```python
from build123d import *

# Parameters (mm, degrees)
PROFILE_EXTRUDE_DEPTH               = 23
PROFILE_EXTRUDE_DEPTH_BACK          = 23
PROFILE_SHELL_T                     = -3
CUFF_JOINT_PIN_SKETCH_R             = 7.5
CUFF_JOIN_PIN_EXTRUDE_DEPTH         = 43
HYDRAULIC_ARM_HOLES_SKETCH_R        = 5
HYDRAULIC_ARM_HOLES_EXTRUDE_1_DEPTH = 3
HYDRAULIC_START                     = -43
HYDRAULIC_ARM_HOLES_SKETCH_2_R      = 5
HYDRAULIC_ARM_HOLES_EXTRUDE_2_DEPTH = 3
HOLES_TABS_FILLET_R                 = 5


with BuildPart() as part:
    # Profile Sketch → Profile Extrude (new, two sides: drawn at the far end of the back side and taken through both)
    with BuildSketch(Plane(origin=(0, 0, 0), x_dir=(0, 0, -1), z_dir=(1, 0, 0)).offset(-PROFILE_EXTRUDE_DEPTH_BACK)):
        with BuildLine():
            Line((-80, 23), (100, 23))
            Line((100, 23), (100, 0))
            ThreePointArc((100, 0), (93.263455967, -16.263455967), (77, -23))
            Line((77, -23), (-100, -23))
            Line((-100, -23), (-100, 3))
            ThreePointArc((-100, 3), (-94.142135624, 17.142135624), (-80, 23))
        make_face()
    extrude(amount=PROFILE_EXTRUDE_DEPTH + PROFILE_EXTRUDE_DEPTH_BACK)

    # Profile Shell
    profile_shell_openings = [part.faces().sort_by_distance(p)[0] for p in [
        (0, 11.5, -100),
        (0, -16.263455967, -93.263455967),
        (0, -23, 11.5),
    ]]
    offset(amount=PROFILE_SHELL_T, openings=profile_shell_openings, kind=Kind.INTERSECTION)

    # Cuff Joint Pin Sketch → Cuff Join Pin Extrude (add)
    with BuildSketch(Plane(origin=(23, 0, 0), x_dir=(0, 0, -1), z_dir=(1, 0, 0))):
        with Locations((77, 0)):
            Circle(CUFF_JOINT_PIN_SKETCH_R)
    extrude(amount=-CUFF_JOIN_PIN_EXTRUDE_DEPTH)

    # Hydraulic Arm Holes Sketch → Hydraulic Arm Holes Extrude 1 (add)
    # profile 1 of 2: a face of its own
    with BuildSketch(Plane(origin=(23, 0, 0), x_dir=(0, 0, -1), z_dir=(1, 0, 0))):
        with BuildLine():
            Line((-100, -23), (-100, -33))
            ThreePointArc((-100, -33), (-90, -43), (-80, -33))
            Line((-80, -33), (-80, -23))
            Line((-80, -23), (-100, -23))
        make_face()
        with Locations((-90, -33)):
            Circle(HYDRAULIC_ARM_HOLES_SKETCH_R, mode=Mode.SUBTRACT)
    # profile 2 of 2: a face of its own
    with BuildSketch(Plane(origin=(23, 0, 0), x_dir=(0, 0, -1), z_dir=(1, 0, 0))):
        with BuildLine():
            Line((-60, -33), (-60, -23))
            Line((-60, -23), (-40, -23))
            Line((-40, -23), (-40, -33))
            ThreePointArc((-40, -33), (-50, -43), (-60, -33))
        make_face()
        with Locations((-50, -33)):
            Circle(HYDRAULIC_ARM_HOLES_SKETCH_R, mode=Mode.SUBTRACT)
    extrude(amount=-HYDRAULIC_ARM_HOLES_EXTRUDE_1_DEPTH)

    # Hydraulic Arm Holes Sketch<2> → Hydraulic Arm Holes Extrude 2 (add)
    # profile 1 of 2: a face of its own
    with BuildSketch(Plane(origin=(23, 0, 0), x_dir=(0, 0, -1), z_dir=(1, 0, 0)).offset(HYDRAULIC_START)):
        with BuildLine():
            Line((-100, -23), (-100, -33))
            ThreePointArc((-100, -33), (-90, -43), (-80, -33))
            Line((-80, -33), (-80, -23))
            Line((-80, -23), (-100, -23))
        make_face()
        with Locations((-90, -33)):
            Circle(HYDRAULIC_ARM_HOLES_SKETCH_2_R, mode=Mode.SUBTRACT)
    # profile 2 of 2: a face of its own
    with BuildSketch(Plane(origin=(23, 0, 0), x_dir=(0, 0, -1), z_dir=(1, 0, 0)).offset(HYDRAULIC_START)):
        with BuildLine():
            Line((-60, -33), (-60, -23))
            Line((-60, -23), (-40, -23))
            Line((-40, -23), (-40, -33))
            ThreePointArc((-40, -33), (-50, -43), (-60, -33))
        make_face()
        with Locations((-50, -33)):
            Circle(HYDRAULIC_ARM_HOLES_SKETCH_2_R, mode=Mode.SUBTRACT)
    extrude(amount=-HYDRAULIC_ARM_HOLES_EXTRUDE_2_DEPTH)

    # Holes Tabs Fillet
    holes_tabs_fillet_edges = [part.edges().sort_by_distance(p)[0] for p in [
        (-21.5, -23, 80),
        (21.5, -23, 40),
        (21.5, -23, 60),
        (21.5, -23, 80),
        (-21.5, -23, 40),
        (-21.5, -23, 60),
    ]]
    fillet(holes_tabs_fillet_edges, radius=HOLES_TABS_FILLET_R)


solid = part.part
```
For this review, take the finished solid that the model builds, in its own axes (mm). A direction names the side the tool comes from. Round coordinates to 2 decimals unless told otherwise and drop trailing zeros. Write each loop counter-clockwise with the first axis right and the second up, starting at its lowest first coordinate (ties: lowest second). Pieces come first, ordered by that corner, then holes. Notation, with made-up numbers: (-15.75, 35.25) -> (20.25, 35.25) arc R34 cw to (20.25, 70.25) -> close; hole circle Ø6 at (-36, 41.5). An arc over 180 degrees is marked (long way). One line per question, with ' | ' between items. Start each with the question number.
1) For pin 1 Ø2 at (x, y) = (-1.5, 5) entering from +Z (3 decimals); pin 2 Ø2 at (x, z) = (9.5, 47) entering from -Y; pin 3 Ø21 at (x, y) = (1, -8) entering from -Z, all flat-tipped, find the tip position at first contact; note any pin that passes through.
2) Add section B-B (x = -18). Write out the cut boundary in (y, z).
3) Machinability: for faces 5 (the cylindrical face through (22, -36, 54)), 6 (the cylindrical face through (21, -25, 61)), 7 (the cylindrical face through (-0.28, 14.89, 92.15)), which of the approach directions +Z, -Z, +X, -X, +Y, -Y give a long, thin tool a straight path to every point of the face, cutting with its end or side? Answer none if there is none.
4) Wall thickness on line 1 along X through (y, z) = (-18.5, 23); line 2 along Y through (x, z) = (21.2, 50); line 3 along Z through (x, y) = (0.5, 0.5): over which ranges is each line inside the solid? List them lowest first.
5) Mouldability with a two-part tool opening along Y and no side actions: class faces 1 (the flat face through (23, -2, 1)), 2 (the cylindrical face through (-0.322, 16.986, 94.297)), 3 (the cylindrical face through (-21.479, -34.915, 85.381)), 4 (the cylindrical face through (21, -24, 38)) as +Y half, -Y half, draft (parallel to the pull), parting line (faces both ways), or undercut.
6) Add section A-A (y = -25). Write out the cut boundary in (x, z).
7) Add section D-D (z = 4.5). Write out the cut boundary in (x, y).
8) Add section C-C (z = 50). Write out the cut boundary in (x, y).
Reported:
1) pin 1: stops at z = 99.975 | pin 2: stops at y = 20 | pin 3: stops at z = -84.5
2) outline: (-23, 97) -> (3, 97) arc R17 cw to (20, 80) -> (20, -100) -> (23, -100) -> (23, 80) arc R20 ccw to (3, 100) -> (-23, 100) -> close; circle Ø15 at (0, -77)
3) face 5: +X, -X | face 6: +X, -X, -Y | face 7: -Y
4) line 1: x = -23 to -20, 20 to 23 | line 2: y = -43 to -38, -28 to 23 | line 3: z = -84.48 to -69.52, 97 to 100
5) face 1: draft | face 2: +Y half | face 3: undercut | face 4: -Y half
6) outline: (-23, 39) -> (-20, 39) -> (-20, 61) -> (-23, 61) -> close; (-23, 79) -> (-20, 79) -> (-20, 100) -> (-23, 100) -> close; (20, 39) -> (23, 39) -> (23, 61) -> (20, 61) -> close; (20, 79) -> (23, 79) -> (23, 100) -> (20, 100) -> close
7) outline: (-23, -23) -> (-20, -23) -> (-20, 20) -> (20, 20) -> (20, -23) -> (23, -23) -> (23, 23) -> (-23, 23) -> close
8) outline: (-23, -43) -> (-20, -43) -> (-20, -38) -> (-23, -38) -> close; (-23, -28) -> (-20, -28) -> (-20, 20) -> (20, 20) -> (20, -28) -> (23, -28) -> (23, 23) -> (-23, 23) -> close; (20, -43) -> (23, -43) -> (23, -38) -> (20, -38) -> close
